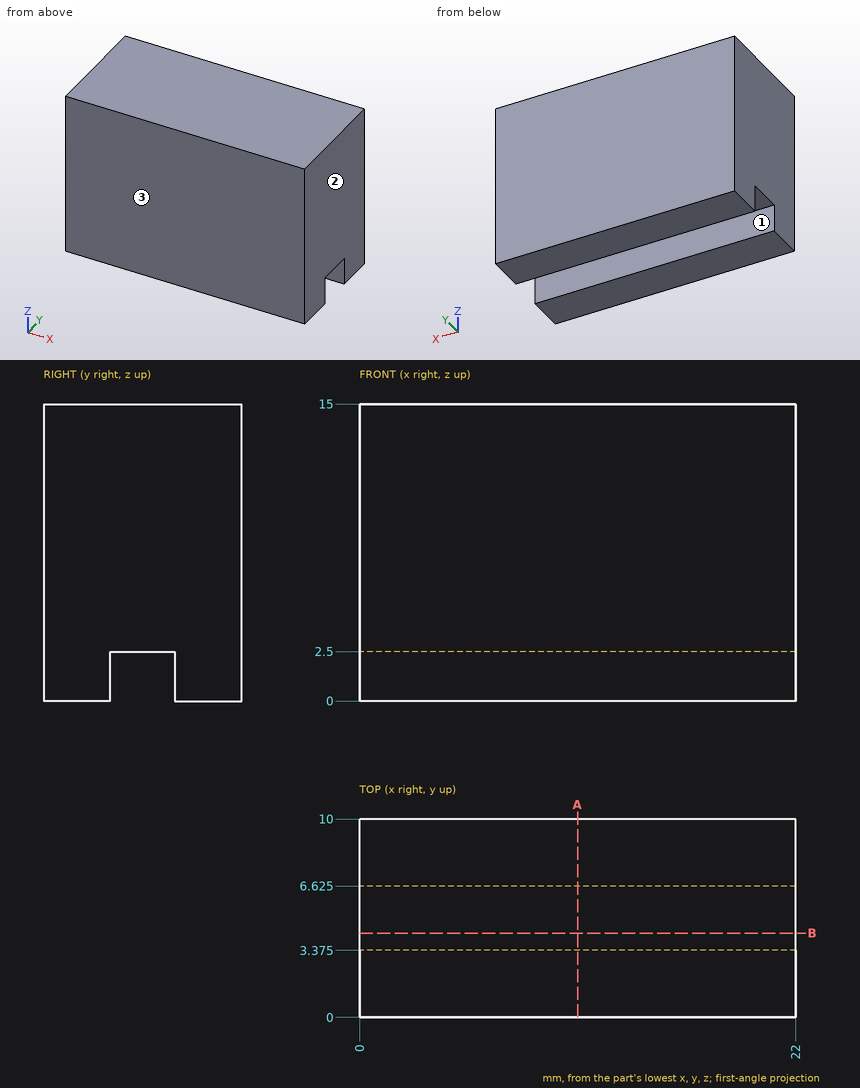
The figure shows three views and two pictorial views of one solid part (mm, origin at its lowest corner). Answer the questions. Coordinates: 2 decimals unless noted, no trailing zeros. Loops run counter-clockwise (first coordinate to the right, second up) from the corner with the lowest first, then second, coordinate; pieces in that order, holes last. Notation, with made-up numbers: (-27.75, 77.25) -> (-5.75, 77.25) arc R12 ccw to (-5.75, 90.25) -> close; hole circle Ø6 at (-15, 28). An arc over 180 degrees is marked (long way). Return JSON: item names as keys, results as strings. Group by question number.
(1) A cutting plane is placed at B-B on y = 4.25. Write down the section's boundary in (x, z), and give its area (3 significant figures).
(2) Given pin 1 Ø1.6 at (x, y) = (6, 5) entering from -Z, flat-ended and moving along its own axis, determine where the tip first touches the part or whether it passes through.
(3) Determine the mould class of the marked faces 1, 2 and 3 for opening direction Y: released by +Y, released by -Y, zero draft, split by the parting line, or undercut.
(4) A cutting plane is placed at A-A on x = 11. Write down the section's boundary in (y, z) (3 decimals).
(5) Find the intervals of material crossed by probe 1 along Y at (x, z) = (4.5, 1.5) (3 decimals); probe 2 along Z at (x, y) = (9, 3.5), in increasing order. Write a range as from..to.
The answers:
{
 "1": {"outline": "(0, 2.5) -> (22, 2.5) -> (22, 15) -> (0, 15) -> close", "area": "275 mm^2"},
 "2": {"pin 1": "stops at z = 2.5"},
 "3": {"face 1": "undercut", "face 2": "zero draft", "face 3": "released by -Y"},
 "4": {"outline": "(0, 0) -> (3.375, 0) -> (3.375, 2.5) -> (6.625, 2.5) -> (6.625, 0) -> (10, 0) -> (10, 15) -> (0, 15) -> close"},
 "5": {"probe 1": "y = 0..3.375, 6.625..10", "probe 2": "z = 2.5..15"}
}
